```python
from build123d import *

# Parameters (mm, degrees)
F1_DEPTH  = 150
F2_DEPTH  = 10
F3_DEPTH  = 20
F4_DEPTH  = 30
F5_DEPTH  = 40
F6_DEPTH  = 50
F7_DEPTH  = 60
F8_DEPTH  = 70
F9_DEPTH  = 80
F10_DEPTH = 90
F11_DEPTH = 100
F12_DEPTH = 110
F13_DEPTH = 120
F14_DEPTH = 130
F15_DEPTH = 140
F16_DEPTH = 150


with BuildPart() as f1:
    # F0 (on Top) → F1 (new body)
    with BuildSketch(Plane.XY):
        with BuildLine():
            ThreePointArc((34.257955, -15.252624), (36.680535, -7.796688), (37.5, 0))
            ThreePointArc((37.5, 0), (36.680535, 7.796688), (34.257955, 15.252624))
            ThreePointArc((34.257955, 15.252624), (30.338137, 22.041947), (25.092398, 27.867931))
            ThreePointArc((25.092398, 27.867931), (18.75, 32.475953), (11.588137, 35.664619))
            ThreePointArc((11.588137, 35.664619), (3.919817, 37.294571), (-3.919817, 37.294571))
            ThreePointArc((-3.919817, 37.294571), (-11.588137, 35.664619), (-18.75, 32.475953))
            ThreePointArc((-18.75, 32.475953), (-25.092398, 27.867931), (-30.338137, 22.041947))
            ThreePointArc((-30.338137, 22.041947), (-34.257955, 15.252624), (-36.680535, 7.796688))
            ThreePointArc((-36.680535, 7.796688), (-37.5, 0), (-36.680535, -7.796688))
            ThreePointArc((-36.680535, -7.796688), (-34.257955, -15.252624), (-30.338137, -22.041947))
            ThreePointArc((-30.338137, -22.041947), (-25.092398, -27.867931), (-18.75, -32.475953))
            ThreePointArc((-18.75, -32.475953), (-11.588137, -35.664619), (-3.919817, -37.294571))
            ThreePointArc((-3.919817, -37.294571), (3.919817, -37.294571), (11.588137, -35.664619))
            ThreePointArc((11.588137, -35.664619), (18.75, -32.475953), (25.092398, -27.867931))
            ThreePointArc((25.092398, -27.867931), (30.338137, -22.041947), (34.257955, -15.252624))
        make_face()
    extrude(amount=F1_DEPTH)

    # F0 (on Top) → F2 (join)
    with BuildSketch(Plane.XY):
        with BuildLine():
            ThreePointArc((-7.839635, -74.589142), (7.839635, -74.589142), (23.176275, -71.329239))
            Line((23.176275, -71.329239), (11.588137, -35.664619))
            ThreePointArc((11.588137, -35.664619), (3.919817, -37.294571), (-3.919817, -37.294571))
            Line((-3.919817, -37.294571), (-7.839635, -74.589142))
        make_face()
    extrude(amount=F2_DEPTH)

    # F0 (on Top) → F3 (join)
    with BuildSketch(Plane.XY):
        with BuildLine():
            ThreePointArc((23.176275, -71.329239), (37.5, -64.951905), (50.184795, -55.735862))
            Line((50.184795, -55.735862), (25.092398, -27.867931))
            ThreePointArc((25.092398, -27.867931), (18.75, -32.475953), (11.588137, -35.664619))
            Line((11.588137, -35.664619), (23.176275, -71.329239))
        make_face()
    extrude(amount=F3_DEPTH)

    # F0 (on Top) → F4 (join)
    with BuildSketch(Plane.XY):
        with BuildLine():
            ThreePointArc((50.184795, -55.735862), (60.676275, -44.083894), (68.515909, -30.505248))
            Line((68.515909, -30.505248), (34.257955, -15.252624))
            ThreePointArc((34.257955, -15.252624), (30.338137, -22.041947), (25.092398, -27.867931))
            Line((25.092398, -27.867931), (50.184795, -55.735862))
        make_face()
    extrude(amount=F4_DEPTH)

    # F0 (on Top) → F5 (join)
    with BuildSketch(Plane.XY):
        with BuildLine():
            ThreePointArc((68.515909, -30.505248), (73.36107, -15.593377), (75, 0))
            Line((75, 0), (37.5, 0))
            ThreePointArc((37.5, 0), (36.680535, -7.796688), (34.257955, -15.252624))
            Line((34.257955, -15.252624), (68.515909, -30.505248))
        make_face()
    extrude(amount=F5_DEPTH)

    # F0 (on Top) → F6 (join)
    with BuildSketch(Plane.XY):
        with BuildLine():
            Line((37.5, 0), (75, 0))
            ThreePointArc((75, 0), (73.36107, 15.593377), (68.515909, 30.505248))
            Line((68.515909, 30.505248), (34.257955, 15.252624))
            ThreePointArc((34.257955, 15.252624), (36.680535, 7.796688), (37.5, 0))
        make_face()
    extrude(amount=F6_DEPTH)

    # F0 (on Top) → F7 (join)
    with BuildSketch(Plane.XY):
        with BuildLine():
            Line((34.257955, 15.252624), (68.515909, 30.505248))
            ThreePointArc((68.515909, 30.505248), (60.676275, 44.083894), (50.184795, 55.735862))
            Line((50.184795, 55.735862), (25.092398, 27.867931))
            ThreePointArc((25.092398, 27.867931), (30.338137, 22.041947), (34.257955, 15.252624))
        make_face()
    extrude(amount=F7_DEPTH)

    # F0 (on Top) → F8 (join)
    with BuildSketch(Plane.XY):
        with BuildLine():
            Line((25.092398, 27.867931), (50.184795, 55.735862))
            ThreePointArc((50.184795, 55.735862), (37.5, 64.951905), (23.176275, 71.329239))
            Line((23.176275, 71.329239), (11.588137, 35.664619))
            ThreePointArc((11.588137, 35.664619), (18.75, 32.475953), (25.092398, 27.867931))
        make_face()
    extrude(amount=F8_DEPTH)

    # F0 (on Top) → F9 (join)
    with BuildSketch(Plane.XY):
        with BuildLine():
            Line((11.588137, 35.664619), (23.176275, 71.329239))
            ThreePointArc((23.176275, 71.329239), (7.839635, 74.589142), (-7.839635, 74.589142))
            Line((-7.839635, 74.589142), (-3.919817, 37.294571))
            ThreePointArc((-3.919817, 37.294571), (3.919817, 37.294571), (11.588137, 35.664619))
        make_face()
    extrude(amount=F9_DEPTH)

    # F0 (on Top) → F10 (join)
    with BuildSketch(Plane.XY):
        with BuildLine():
            Line((-3.919817, 37.294571), (-7.839635, 74.589142))
            ThreePointArc((-7.839635, 74.589142), (-23.176275, 71.329239), (-37.5, 64.951905))
            Line((-37.5, 64.951905), (-18.75, 32.475953))
            ThreePointArc((-18.75, 32.475953), (-11.588137, 35.664619), (-3.919817, 37.294571))
        make_face()
    extrude(amount=F10_DEPTH)

    # F0 (on Top) → F11 (join)
    with BuildSketch(Plane.XY):
        with BuildLine():
            Line((-18.75, 32.475953), (-37.5, 64.951905))
            ThreePointArc((-37.5, 64.951905), (-50.184795, 55.735862), (-60.676275, 44.083894))
            Line((-60.676275, 44.083894), (-30.338137, 22.041947))
            ThreePointArc((-30.338137, 22.041947), (-25.092398, 27.867931), (-18.75, 32.475953))
        make_face()
    extrude(amount=F11_DEPTH)

    # F0 (on Top) → F12 (join)
    with BuildSketch(Plane.XY):
        with BuildLine():
            Line((-30.338137, 22.041947), (-60.676275, 44.083894))
            ThreePointArc((-60.676275, 44.083894), (-68.515909, 30.505248), (-73.36107, 15.593377))
            Line((-73.36107, 15.593377), (-36.680535, 7.796688))
            ThreePointArc((-36.680535, 7.796688), (-34.257955, 15.252624), (-30.338137, 22.041947))
        make_face()
    extrude(amount=F12_DEPTH)

    # F0 (on Top) → F13 (join)
    with BuildSketch(Plane.XY):
        with BuildLine():
            Line((-36.680535, 7.796688), (-73.36107, 15.593377))
            ThreePointArc((-73.36107, 15.593377), (-75, 0), (-73.36107, -15.593377))
            Line((-73.36107, -15.593377), (-36.680535, -7.796688))
            ThreePointArc((-36.680535, -7.796688), (-37.5, 0), (-36.680535, 7.796688))
        make_face()
    extrude(amount=F13_DEPTH)

    # F0 (on Top) → F14 (join)
    with BuildSketch(Plane.XY):
        with BuildLine():
            ThreePointArc((-73.36107, -15.593377), (-68.515909, -30.505248), (-60.676275, -44.083894))
            Line((-60.676275, -44.083894), (-30.338137, -22.041947))
            ThreePointArc((-30.338137, -22.041947), (-34.257955, -15.252624), (-36.680535, -7.796688))
            Line((-36.680535, -7.796688), (-73.36107, -15.593377))
        make_face()
    extrude(amount=F14_DEPTH)

    # F0 (on Top) → F15 (join)
    with BuildSketch(Plane.XY):
        with BuildLine():
            ThreePointArc((-60.676275, -44.083894), (-50.184795, -55.735862), (-37.5, -64.951905))
            Line((-37.5, -64.951905), (-18.75, -32.475953))
            ThreePointArc((-18.75, -32.475953), (-25.092398, -27.867931), (-30.338137, -22.041947))
            Line((-30.338137, -22.041947), (-60.676275, -44.083894))
        make_face()
    extrude(amount=F15_DEPTH)

    # F0 (on Top) → F16 (join)
    with BuildSketch(Plane.XY):
        with BuildLine():
            ThreePointArc((-37.5, -64.951905), (-23.176275, -71.329239), (-7.839635, -74.589142))
            Line((-7.839635, -74.589142), (-3.919817, -37.294571))
            ThreePointArc((-3.919817, -37.294571), (-11.588137, -35.664619), (-18.75, -32.475953))
            Line((-18.75, -32.475953), (-37.5, -64.951905))
        make_face()
    extrude(amount=F16_DEPTH)


solid = f1.part
```
Input: part model. Units: mm. Frame: model coordinates. A direction names the side the tool comes from. Coordinates: 2 decimals unless noted, no trailing zeros. Loops run counter-clockwise (first coordinate to the right, second up) from the corner with the lowest first, then second, coordinate; pieces in that order, holes last. Notation, with made-up numbers: M -9,6.5 L 35,6.5 A22 ccw 35,21.5 Z; hole C -4.5,71.5 d2. An arc over 180 degrees is marked long. Use a Markdown table: item, result. Add a question column.
1) Section A-A, the plane z = 103. Return the cut outline in (x, y), plus the area to 3 significant figures.
2) Section D-D, the plane z = 27. Return the cut outline in (x, y), plus the area to 3 significant figures.
3) Section C-C, the plane x = -58. Return the cut outline in (y, z).
4) Draft query along Y for faces 5 (the flat face through (59, -12, 40)), 6 (the cylindrical face through (-37.5, 0.1, 134.8)), 7 (the flat face through (-54.76, 11.64, 114.93)). Return one class per face: +Y half, -Y half, draft (parallel to the pull), parting line (faces both ways), or undercut.
5) Line query: L1, parallel to Z at x = -43, y = 6; L2, parallel to Z at x = 48, y = -18; L3, parallel to Y at x = 31.5, z = 67. Output: solid intervals per line, ascending. Write a range as from..to.
6) Set-up query: faces 1 (the flat face through (-40, 44, 100)), 2 (the flat face through (-40, -43, 140)), 3 (the flat face through (37.463, -41.607, 24.93)), 4 (the flat face through (-5.852, 55.681, 84.93)). Return all of +Z, -Z, +X, -X, +Y, -Y with unobstructed straight access to the full face (end or side cutting, diameter ignored); none if empty.
7) Section B-B, the plane y = -40. Return the cut outline in (x, z).
8) Pin query (flat end, axial travel): P1, Ø11.5, axis at x = 34.5, y = 46, coming from the +Z side; P2, Ø3, axis at x = -54.5, z = 31, coming from the -Y side; P3, Ø4, axis at x = 6.5, z = 128, coming from the -Y side. Return the tip coordinate at first contact, or that it passes through.
Answer below:
| question | item | result |
|---|---|---|
| 1 | outline | M -73.36,-15.59 A75 ccw -60.68,-44.08 A75 ccw -37.5,-64.95 A75 ccw -7.84,-74.59 L -3.92,-37.29 A37.5 ccw 11.59,-35.66 A37.5 ccw 25.09,-27.87 A37.5 ccw 34.26,-15.25 A37.5 ccw 37.5,0 A37.5 ccw 34.26,15.25 A37.5 ccw 25.09,27.87 A37.5 ccw 11.59,35.66 A37.5 ccw -3.92,37.29 A37.5 ccw -18.75,32.48 A37.5 ccw -30.34,22.04 L -60.68,44.08 A75 ccw -73.36,15.59 A75 ccw Z |
| 1 | area | 8,840 mm2 |
| 2 | outline | M -73.36,-15.59 A75 ccw -60.68,-44.08 A75 ccw -37.5,-64.95 A75 ccw -7.84,-74.59 L -3.92,-37.29 A37.5 ccw 11.59,-35.66 A37.5 ccw 25.09,-27.87 L 50.18,-55.74 A75 ccw 68.52,-30.51 A75 ccw 75,0 A75 ccw 68.52,30.51 A75 ccw 50.18,55.74 A75 ccw 23.18,71.33 A75 ccw -7.84,74.59 A75 ccw -37.5,64.95 A75 ccw -60.68,44.08 A75 ccw -73.36,15.59 A75 ccw Z |
| 2 | area | 15,900 mm2 |
| 3 | outline | M -47.55,0 L 47.55,0 L 47.55,100 L 42.14,100 L 42.14,110 L 12.33,110 L 12.33,120 L -12.33,120 L -12.33,130 L -42.14,130 L -42.14,140 L -47.55,140 Z |
| 4 | face 5 | draft |
| 4 | face 6 | undercut |
| 4 | face 7 | +Y half |
| 5 | L1 | 0..120 |
| 5 | L2 | 0..40 |
| 5 | L3 | -20.35..20.35, 34.98..68.06 |
| 6 | face 1 | +Z, +Y |
| 6 | face 2 | +Z, -X |
| 6 | face 3 | +Z, -Y |
| 6 | face 4 | +Z, +X, +Y |
| 7 | outline | M -63.44,0 L 63.44,0 L 63.44,30 L 36.02,30 L 36.02,20 L 13,20 L 13,10 L -4.2,10 L -4.2,150 L -23.09,150 L -23.09,140 L -55.06,140 L -55.06,130 L -63.44,130 Z |
| 8 | P1 | z = 70 |
| 8 | P2 | y = -53.07 |
| 8 | P3 | y = -37.23 |
